Check sheet for the drawn part. Datum: minimum x, y, z corner. Units: mm. Round coordinates to 2 decimals unless told otherwise and drop trailing zeros. Order: outer loops, then holes, each group sorted by start corner. A loop starts at its lowest first (then second) coordinate and runs counter-clockwise, first axis right, second up. Notation, with made-up numbers: M 40,62.5 L 63,62.5 A22 ccw 63,92.5 Z; hole C 50,3 d8. An arc over 180 degrees is marked long. Answer as a JSON object with one key per item and string values. Group by question number.
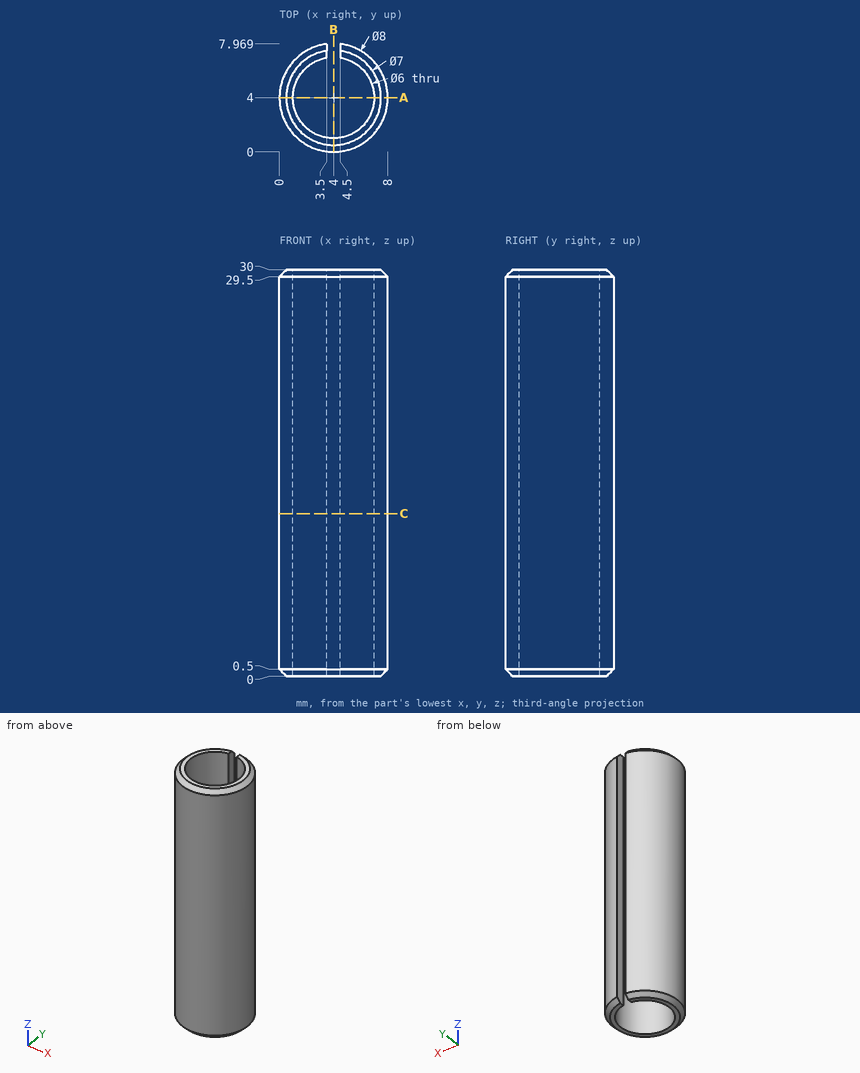
1) Sectioned sample at C-C (z = 12). Record the boundary of the cut face in (x, y).
2) Sectioned sample at A-A (y = 4). Record the boundary of the cut face in (x, z).
3) Go/stop test with flat-tipped pins: P1, Ø0.8, axis at y = 7.5, z = 11.5, coming from the +X side; P2, Ø4, axis at y = 1.5, z = 25, coming from the -X side; P3, Ø3.5, axis at x = 4, y = 4, coming from the +Z side; P4, Ø1, axis at x = 6.5, z = 14.5, coming from the -Y side (1 decimal). Record where each tip stops, or that it passes through.
4) Thickness scan on line 1 along X through (y, z) = (4, 7); line 2 along Y through (x, z) = (3.25, 13) (1 decimal); line 3 along Y through (x, z) = (5.5, 15.5). Record the ranges inside material, lowest first. Write a range as [from, to].
5) Sectioned sample at B-B (x = 4). Record the boundary of the cut face in (y, z).
Final values:
{
 "1": {"outline": "M 3.5,6.96 L 3.5,7.97 A4 ccw long 4.5,7.97 L 4.5,6.96 A3 cw long Z"},
 "2": {"outline": "M 0,0.5 L 0.5,0 L 1,0 L 1,30 L 0.5,30 L 0,29.5 Z; M 7,0 L 7.5,0 L 8,0.5 L 8,29.5 L 7.5,30 L 7,30 Z"},
 "3": {"P1": "stops at x = 6.53", "P2": "stops at x = 0.03", "P3": "passes through", "P4": "stops at y = 0.5"},
 "4": {"line 1": "x = [0, 1], [7, 8]", "line 2": "y = [0.1, 1.1], [6.9, 7.9]", "line 3": "y = [0.29, 1.4], [6.6, 7.71]"},
 "5": {"outline": "M 0,0.5 L 0.5,0 L 1,0 L 1,30 L 0.5,30 L 0,29.5 Z"}
}
